```python
from build123d import *

# Parameters (mm, degrees)
BOSS_EXTRUDE1_DEPTH = 4
SKETCH2_W           = 5
SKETCH2_H           = 10
BOSS_EXTRUDE2_DEPTH = 20
SKETCH3_R           = 2.65
CUT_EXTRUDE1_DEPTH  = 20
FILLET1_R           = 5
SKETCH4_W           = 5
SKETCH4_H           = 10
BOSS_EXTRUDE3_DEPTH = 20
SKETCH5_R           = 2.65
CUT_EXTRUDE2_DEPTH  = 20
FILLET2_R           = 5
SKETCH6_W           = 28
SKETCH6_H           = 6
BOSS_EXTRUDE4_DEPTH = 20
SKETCH7_R           = 5.1
CUT_EXTRUDE3_DEPTH  = 3.2
FILLET3_R           = 14
FILLET4_R           = 5


# Some blends are built 0.0001 mm under size
with BuildPart() as part:
    # Sketch1 → Boss-Extrude1 (new body)
    with BuildSketch(Plane.XY):
        Polygon((0, 0), (885, 0), (885, 55), (820, 120), (0, 120), align=None)
    extrude(amount=BOSS_EXTRUDE1_DEPTH)

    # Sketch2 → Boss-Extrude2 (add)
    with BuildSketch(Plane(origin=(0, 0, 0), x_dir=(-1, 0, 0), z_dir=(0, 0, -1))):
        with Locations((-22.5, 90)):
            Rectangle(SKETCH2_W, SKETCH2_H)
        with Locations((-22.5, 35)):
            Rectangle(SKETCH2_W, SKETCH2_H)
    extrude(amount=BOSS_EXTRUDE2_DEPTH)

    # Sketch3 → Cut-Extrude1 (cut)
    with BuildSketch(Plane(origin=(25, 0, 0), x_dir=(0, 0, -1), z_dir=(1, 0, 0))):
        with Locations(Location((10, 90, 0), (0, 0, 90))):
            Circle(SKETCH3_R)
        with Locations(Location((10, 35, 0), (0, 0, 90))):
            Circle(SKETCH3_R)
    extrude(amount=-CUT_EXTRUDE1_DEPTH, mode=Mode.SUBTRACT)

    # Fillet1
    fillet1_edges = [part.edges().sort_by_distance(p)[0] for p in [
        (22.5, 30, -20),
        (22.5, 40, -20),
        (22.5, 85, -20),
        (22.5, 95, -20),
    ]]
    fillet(fillet1_edges, radius=FILLET1_R - 0.0001)  # a hair under: the kernel refuses the full size

    # Sketch4 → Boss-Extrude3 (add)
    with BuildSketch(Plane(origin=(0, 0, 0), x_dir=(-1, 0, 0), z_dir=(0, 0, -1))):
        with Locations((-862.5, 30)):
            Rectangle(SKETCH4_W, SKETCH4_H)
    extrude(amount=BOSS_EXTRUDE3_DEPTH)

    # Sketch5 → Cut-Extrude2 (cut)
    with BuildSketch(Plane(origin=(865, 0, 0), x_dir=(0, 0, -1), z_dir=(1, 0, 0))):
        with Locations((10, 30)):
            Circle(SKETCH5_R)
    extrude(amount=-CUT_EXTRUDE2_DEPTH, mode=Mode.SUBTRACT)

    # Fillet2
    fillet2_edges = [part.edges().sort_by_distance(p)[0] for p in [
        (862.5, 25, -20),
        (862.5, 35, -20),
    ]]
    fillet(fillet2_edges, radius=FILLET2_R - 0.0001)  # a hair under: the kernel refuses the full size

    # Sketch6 → Boss-Extrude4 (add)
    with BuildSketch(Plane(origin=(0, 0, 0), x_dir=(-1, 0, 0), z_dir=(0, 0, -1))):
        with Locations((-806, 117)):
            Rectangle(SKETCH6_W, SKETCH6_H)
    extrude(amount=BOSS_EXTRUDE4_DEPTH)

    # Sketch7 → Cut-Extrude3 (cut)
    with BuildSketch(Plane(origin=(0, 120, 0), x_dir=(1, 0, 0), z_dir=(0, 1, 0))):
        with Locations(Location((806, 10, 0), (0, 0, 180))):
            Circle(SKETCH7_R)
    extrude(amount=-CUT_EXTRUDE3_DEPTH, mode=Mode.SUBTRACT)

    # Fillet3
    fillet3_edges = [part.edges().sort_by_distance(p)[0] for p in [
        (792, 117, -20),
        (820, 117, -20),
    ]]
    fillet(fillet3_edges, radius=FILLET3_R - 0.0001)  # a hair under: the kernel refuses the full size

    # Fillet4
    # the kernel refuses this fillet: 5 mm, written as the material it takes off along each edge
    with BuildSketch(Plane(origin=(-12.247448714, 0, 4), x_dir=(0, 1, 0), z_dir=(1, 0, 0))) as fillet4_piece_1:
        with BuildLine():
            CenterArc((4.898979486, -5), FILLET4_R, 90, 78.463040967)
            Line((0, -4), (-0.09797959, -3.98))
            ThreePointArc((-0.09797959, -3.98), (-0.1, -2), (-0.1, 0))
            Line((-0.1, 0), (0, 0.1))
            Line((0, 0.1), (4.898979486, 0.1))
            Line((4.898979486, 0.1), (4.898979486, 0))
        make_face()
    extrude(amount=909.494897428, mode=Mode.SUBTRACT)


solid = part.part
```
Geometry check sheet. Reference: the model listing, model coordinates, mm. A direction names the side the tool comes from. Round coordinates to 2 decimals unless told otherwise and drop trailing zeros. Loops run counter-clockwise (first coordinate to the right, second up) from the corner with the lowest first, then second, coordinate; pieces in that order, holes last. Notation, with made-up numbers: M -29,71 L 10,71 A35 cw 10,105 Z; hole C 21,5 d9. An arc over 180 degrees is marked long. Return JSON: item names as keys, results as strings. Group by question number.
(1) Scan lines: line 1 along Y through (x, z) = (862.4, -10); line 2 along Z through (x, y) = (22.9, 35); line 3 along Z through (x, y) = (597.5, 32). Record each from-to range of solid material in increasing order. Write a range as [from, to].
(2) Set-up check for faces 1 (the face through (853, 87, 2)), 2 (the face through (806, 114, -8)): record each of +Z, -Z, +X, -X, +Y, -Y from which the full face is reachable in a straight line by a thin tool's end or side.
(3) Section check A-A, the plane x = 674.5. Enter the section's corners in (y, z).
(4) Go/stop test with flat-tipped pins: pin 1 (4 mm diameter, centred on x = 862.5, z = -6, fed in from +Y); pin 2 (5 mm diameter, centred on y = 43.5, z = -3.5, fed in from -X); pin 3 (8 mm diameter, centred on y = 28, z = -14, fed in from +X); pin 4 (2.5 mm diameter, centred on x = 23, z = -8.5, fed in from -Y). Record where each tip stops, or that it passes through.
Data:
{
 "1": {"line 1": "[25, 27.35], [32.65, 35]", "line 2": "[-20, -12.65], [-7.35, 4]", "line 3": "[0, 4]"},
 "2": {"face 1": "+Z, -Z, +X, +Y", "face 2": "-Z, +X, -X, -Y"},
 "3": {"outline": "M 0,0 L 120,0 L 120,4 L 4.9,4 A5 ccw Z"},
 "4": {"pin 1": "y = 35", "pin 2": "through", "pin 3": "x = 865", "pin 4": "y = 30"}
}
